```python
from build123d import *

# Parameters (mm, degrees)
BOSS_EXTRUDE1_DEPTH = 19
SKETCH3_R           = 1.5
CUT_EXTRUDE2_DEPTH  = 18
SKETCH2_R           = 5.25
CUT_EXTRUDE4_DEPTH  = 10
SKETCH4_R           = 3
CUT_EXTRUDE5_DEPTH  = 10


with BuildPart() as part:
    # Sketch1 → Boss-Extrude1 (new, symmetric)
    with BuildSketch(Plane.XY):
        with BuildLine():
            Line((21.027756377, 6), (21.027756377, 18))
            Line((21.027756377, 18), (43, 18))
            Line((43, 18), (43, 28))
            Line((43, 28), (22.627416998, 28))
            ThreePointArc((22.627416998, 28), (0, 36), (-22.627416998, 28))
            Line((-22.627416998, 28), (-43, 28))
            Line((-43, 28), (-43, 18))
            Line((-43, 18), (-21.027756377, 18))
            Line((-21.027756377, 18), (-21.027756377, 6))
            Line((-21.027756377, 6), (-18.027756377, 6))
            ThreePointArc((-18.027756377, 6), (0, 19), (18.027756377, 6))
            Line((18.027756377, 6), (21.027756377, 6))
        make_face()
    extrude(amount=BOSS_EXTRUDE1_DEPTH, both=True)

    # Sketch3 → Cut-Extrude2 (cut)
    with BuildSketch(Plane(origin=(0, 36, 0), x_dir=(1, 0, 0), z_dir=(0, 1, 0))):
        with Locations(Location((0, 0, 0), (0, 0, 270))):
            Circle(SKETCH3_R)
    extrude(amount=-CUT_EXTRUDE2_DEPTH, mode=Mode.SUBTRACT)

    # Sketch2 → Cut-Extrude4 (cut)
    with BuildSketch(Plane(origin=(0, 28, 0), x_dir=(1, 0, 0), z_dir=(0, 1, 0))):
        with Locations(Location((30, 0, 0), (0, 0, 270))):
            Circle(SKETCH2_R)
        with Locations(Location((-31, 0, 0), (0, 0, 270))):
            Circle(SKETCH2_R)
    extrude(amount=-CUT_EXTRUDE4_DEPTH, mode=Mode.SUBTRACT)

    # Sketch4 → Cut-Extrude5 (cut)
    with BuildSketch(Plane(origin=(0, 36, 0), x_dir=(1, 0, 0), z_dir=(0, 1, 0))):
        with Locations(Location((0, 0, 0), (0, 0, 270))):
            Circle(SKETCH4_R)
    extrude(amount=-CUT_EXTRUDE5_DEPTH, mode=Mode.SUBTRACT)


solid = part.part
```
Check sheet for the modelled part. Datum: model origin and axes. Units: mm. A direction names the side the tool comes from. Give positions to 0.01 mm unless a question says otherwise; leave off trailing zeros. Write each loop counter-clockwise with the first axis right and the second up, starting at its lowest first coordinate (ties: lowest second). Pieces come first, ordered by that corner, then holes.
Item 1: Draft check along Z on faces 5 (the face through (37, 28, 0)), 6 (the face through (34.43, 23.07, 2.82)), 7 (the face through (-1, 25, 19)). Enter one of: released by +Z, released by -Z, zero draft, split by the parting line, or undercut.
Item 2: Cross-section at C-C (y = 24). Enter the section's corners in (x, z), and give its area (3 significant figures).
Item 3: Scan lines: L1, parallel to X at y = 24, z = 0; L2, parallel to X at y = 8, z = -10.5; L3, parallel to Y at x = -39, z = 8.5. Record each from-to range of solid material in increasing order.
Item 4: Cross-section at D-D (z = 12.5). Enter the section's corners in (x, y), and give its area (3 significant figures).
Item 5: Cross-section at A-A (x = 0). Enter the section's corners in (y, z), and give its area (3 significant figures).
Item 6: Cross-section at B-B (z = 0). Enter the section's corners in (x, y), and give its area (3 significant figures).
Item 7: Gauge pin test, flat ends, axial feed: pin 1 (10 mm diameter, centred on x = -34, z = 6, fed in from +Y); pin 2 (12 mm diameter, centred on y = 11, z = 10, fed in from +X); pin 3 (6 mm diameter, centred on x = 18.5, z = 6.5, fed in from +Y); pin 4 (10 mm diameter, centred on x = -1, z = 15, fed in from +Y). Record the tip position at first contact, or that the pin passes through.
Item 8: Access from +Z, -Z, +X, -X, +Y, -Y to the whole of each face (thin tool, end or side, straight path). Record for faces 1 (the face through (-37, 18, 0)), 2 (the face through (-37, 28, 0)), 3 (the face through (37, 18, 0)), 4 (the face through (0.9, 31.07, 2.86)).
Report:
1. face 5: zero draft
1. face 6: undercut
1. face 7: released by +Z
2. outline: (-43, -19) - (43, -19) - (43, 19) - (-43, 19) - close; hole circle Ø10.5 at (-31, 0); hole circle Ø3 at (0, 0); hole circle Ø10.5 at (30, 0)
2. area: 3,090 mm2
3. L1: x = -43 to -36.25, -25.75 to -1.5, 1.5 to 24.75, 35.25 to 43
3. L2: x = -21.03 to -17.23, 17.23 to 21.03
3. L3: y = 18 to 28
4. outline: (-43, 18) - (-21.03, 18) - (-21.03, 6) - (-18.03, 6) arc R19 cw to (18.03, 6) - (21.03, 6) - (21.03, 18) - (43, 18) - (43, 28) - (22.63, 28) arc R36 ccw to (-22.63, 28) - (-43, 28) - close
4. area: 1,270 mm2
5. outline: (19, -19) - (36, -19) - (36, -3) - (26, -3) - (26, -1.5) - (19, -1.5) - close; (19, 1.5) - (26, 1.5) - (26, 3) - (36, 3) - (36, 19) - (19, 19) - close
5. area: 565 mm2
6. outline: (-43, 18) - (-36.25, 18) - (-36.25, 28) - (-43, 28) - close; (-25.75, 18) - (-21.03, 18) - (-21.03, 6) - (-18.03, 6) arc R19 cw to (-1.5, 18.94) - (-1.5, 26) - (-3, 26) - (-3, 35.87) arc R36 ccw to (-22.63, 28) - (-25.75, 28) - close; (1.5, 18.94) arc R19 cw to (18.03, 6) - (21.03, 6) - (21.03, 18) - (24.75, 18) - (24.75, 28) - (22.63, 28) arc R36 ccw to (3, 35.87) - (3, 26) - (1.5, 26) - close; (35.25, 18) - (43, 18) - (43, 28) - (35.25, 28) - close
6. area: 978 mm2
7. pin 1: stops at y = 28
7. pin 2: stops at x = 21.03
7. pin 3: stops at y = 32.49
7. pin 4: stops at y = 36
8. face 1: +Z, -Z, -X, -Y
8. face 2: +Z, -Z, -X, +Y
8. face 3: +Z, -Z, +X, -Y
8. face 4: +Y
